from build123d import *

# Parameters (mm, degrees)
SKETCH3_R           = 11
SKETCH3_R_2         = 5
BOSS_EXTRUDE1_DEPTH = 5.95
SKETCH4_R           = 9.75
SKETCH4_R_2         = 6.75
CUT_EXTRUDE1_DEPTH  = 0.25


with BuildPart() as part:
    # Sketch3 → Boss-Extrude1 (new body)
    with BuildSketch(Plane.XY):
        Circle(SKETCH3_R)
        Circle(SKETCH3_R_2, mode=Mode.SUBTRACT)
    extrude(amount=BOSS_EXTRUDE1_DEPTH)

    # Sketch4 → Cut-Extrude1 (cut)
    with BuildSketch(Plane.XY.offset(5.95)):
        Circle(SKETCH4_R)
        Circle(SKETCH4_R_2, mode=Mode.SUBTRACT)
    cut_extrude1 = extrude(amount=-CUT_EXTRUDE1_DEPTH, mode=Mode.SUBTRACT)

    # Mirror1: Cut-Extrude1 across plane
    add(cut_extrude1.mirror(Plane.XY.offset(2.975)), mode=Mode.SUBTRACT)


solid = part.part
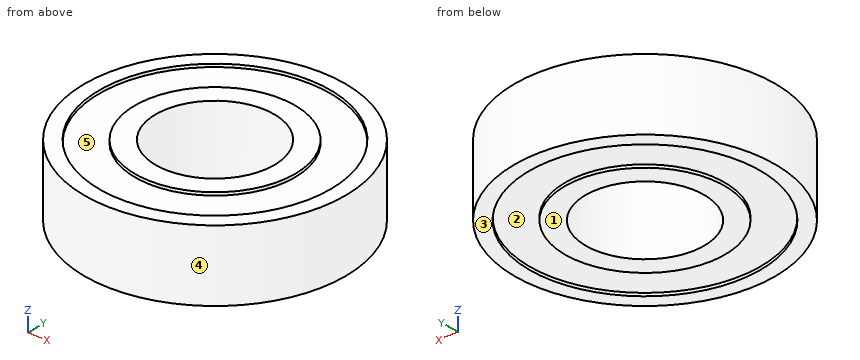
Source: CAD feature listing. Evaluate the final solid. Frame: model axes, mm. Face numbers are marked on the shaded views. A direction names the side the tool comes from. Coordinates: 2 decimals unless noted, no trailing zeros. Loops run counter-clockwise (first coordinate to the right, second up) from the corner with the lowest first, then second, coordinate; pieces in that order, holes last. Notation, with made-up numbers: (1, 64.5) -> (12, 64.5) arc R26 cw to (12, 96.5) -> close; hole circle Ø11 at (82.5, 34.25). An arc over 180 degrees is marked (long way). Answer in a Markdown table with one row per item. Add a question column.
Q1. Pull-direction query (Y, two-part tool) for the marked faces 3, 4 and 5; classes: pulls with the +Y half, pulls with the -Y half, needs draft (parallel to the pull), parting line crosses it, or undercut.
Q2. Section D-D on y = 7.5. Return the cut outline in (x, z), and give its area (3 significant figures).
Q3. Section C-C on z = 1. Return the cut outline in (x, y), and give its area (3 significant figures).
Q4. Contact query for flat-ended pins moving along their axis: pin 1 Ø11.5 at (x, y) = (0, 0) entering from +Z; pin 2 Ø1.5 at (x, z) = (5.5, 5) entering from +Y; pin 3 Ø3 at (x, z) = (-7, 2.5) entering from -Y; pin 4 Ø3 at (y, z) = (2, 1) entering from +X. Output: stop coordinate, or through.
Q5. Section A-A on x = 0. Return the cut outline in (y, z), and give its area (3 significant figures).
Q6. Reachability of the marked faces 1 and 2 from +Z, -Z, +X, -X, +Y, -Y: full face, straight path, thin tool, end or side. Return the list, or none.
Q7. Ray query, line 1 along Y through (x, z) = (0.25, 3.85); line 2 along Y through (x, z) = (0, 0.1); line 3 along Y through (x, z) = (2, 5.1). Return the intervals inside material, ascending.
Computed values:
| question | item | result |
|---|---|---|
| 1 | face 3 | needs draft |
| 1 | face 4 | parting line crosses it |
| 1 | face 5 | undercut |
| 2 | outline | (-8.05, 0) -> (-6.23, 0) -> (-6.23, 0.25) -> (6.23, 0.25) -> (6.23, 0) -> (8.05, 0) -> (8.05, 5.95) -> (6.23, 5.95) -> (6.23, 5.7) -> (-6.23, 5.7) -> (-6.23, 5.95) -> (-8.05, 5.95) -> close |
| 2 | area | 89.5 mm^2 |
| 3 | outline | circle Ø22 at (0, 0); hole circle Ø10 at (0, 0) |
| 3 | area | 302 mm^2 |
| 4 | pin 1 | stops at z = 5.95 |
| 4 | pin 2 | stops at y = 9.92 |
| 4 | pin 3 | stops at y = -9.53 |
| 4 | pin 4 | stops at x = 10.99 |
| 5 | outline | (-11, 0) -> (-9.75, 0) -> (-9.75, 0.25) -> (-6.75, 0.25) -> (-6.75, 0) -> (-5, 0) -> (-5, 5.95) -> (-6.75, 5.95) -> (-6.75, 5.7) -> (-9.75, 5.7) -> (-9.75, 5.95) -> (-11, 5.95) -> close; (5, 0) -> (6.75, 0) -> (6.75, 0.25) -> (9.75, 0.25) -> (9.75, 0) -> (11, 0) -> (11, 5.95) -> (9.75, 5.95) -> (9.75, 5.7) -> (6.75, 5.7) -> (6.75, 5.95) -> (5, 5.95) -> close |
| 5 | area | 68.4 mm^2 |
| 6 | face 1 | -Z, +X, -X, +Y, -Y |
| 6 | face 2 | -Z |
| 7 | line 1 | y = -11 to -4.99, 4.99 to 11 |
| 7 | line 2 | y = -11 to -9.75, -6.75 to -5, 5 to 6.75, 9.75 to 11 |
| 7 | line 3 | y = -10.82 to -4.58, 4.58 to 10.82 |
